```python
from build123d import *

# Parameters (mm, degrees)
SKETCH1_W           = 25.4
SKETCH1_H           = 50.8
SKETCH1_W_2         = 22.2504
SKETCH1_H_2         = 47.6504
BOSS_EXTRUDE1_DEPTH = 406.4
SKETCH2_R           = 14.2875
CUT_EXTRUDE1_DEPTH  = 51.8
SKETCH3_R           = 14.2875
SKETCH3_R_2         = 12.6365
BOSS_EXTRUDE2_DEPTH = 50.8


with BuildPart() as part:
    # Sketch1 → Boss-Extrude1 (new body)
    with BuildSketch(Plane.XY):
        Rectangle(SKETCH1_W, SKETCH1_H)
        Rectangle(SKETCH1_W_2, SKETCH1_H_2, mode=Mode.SUBTRACT)
    extrude(amount=BOSS_EXTRUDE1_DEPTH)

    # Sketch2 → Cut-Extrude1 (cut, through all)
    with BuildSketch(Plane(origin=(0, 25.4, 0), x_dir=(1, 0, 0), z_dir=(0, 1, 0))):
        Circle(SKETCH2_R)
        with Locations((0, -406.4)):
            Circle(SKETCH2_R)
    extrude(amount=-CUT_EXTRUDE1_DEPTH, mode=Mode.SUBTRACT)

    # Sketch3 → Boss-Extrude2 (add)
    with BuildSketch(Plane(origin=(0, 25.4, 0), x_dir=(1, 0, 0), z_dir=(0, 1, 0))):
        Circle(SKETCH3_R)
        Circle(SKETCH3_R_2, mode=Mode.SUBTRACT)
        with Locations((0, -406.4)):
            Circle(SKETCH3_R)
        with Locations((0, -406.4)):
            Circle(SKETCH3_R_2, mode=Mode.SUBTRACT)
    extrude(amount=-BOSS_EXTRUDE2_DEPTH)


solid = part.part
```
The model under review builds one solid part; all positions refer to its coordinate system, in mm. A direction names the side the tool comes from. Coordinates: 2 decimals unless noted, no trailing zeros. Order: outer loops, then holes, each group sorted by start corner. A loop starts at its lowest first (then second) coordinate and runs counter-clockwise, first axis right, second up. Notation, with made-up numbers: (42, -37) -> (76, -37) arc R23 ccw to (76, -18) -> close; hole circle Ø3 at (-39, -38). An arc over 180 degrees is marked (long way). Answer in a Markdown table with one row per item. Add a question column.
Item 1: Clearance check with flat-ended pins moving along their axes: pin 1 (15 mm diameter, centred on y = 12, z = 278.5, fed in from +X); pin 2 (6 mm diameter, centred on x = 11, y = -1.5, fed in from -Z); pin 3 (5 mm diameter, centred on x = -7, y = 8, fed in from -Z). State where each tip first meets the part, or that it passes through.
Item 2: We need section B-B on z = 0. Write out the cut boundary in (x, y).
Item 3: To check wall thickness, follow probe 1 along Z at (x, y) = (0.25, 11.5); probe 2 along Z at (x, y) = (1.25, 1); probe 3 along Y at (x, z) = (-7.75, 317). State the ranges of each line that lie inside material, in increasing order.
Item 4: Machinability: for faces 1 (the flat face through (3, -25.4, 200)), 2 (the flat face through (12.7, 0, 200)), 3 (the flat face through (0, 23.825, 200)), 4 (the flat face through (-12.7, 0, 200)), which of the approach directions +Z, -Z, +X, -X, +Y, -Y give a long, thin tool a straight path to every point of the face, cutting with its end or side? Answer none if there is none.
Item 5: We need section A-A on x = 0. Write out the cut boundary in (y, z), plus the area to 3 significant figures.
Item 6: We need section C-C on y = 18.5. Write out the cut boundary in (x, z) (1 decimal), plus the area to 3 significant figures.
Item 7: Mouldability with a two-part tool opening along Z and no side actions: class faces 5 (the cylindrical face through (-1.65, 0.36, 393.87)), 6 (the flat face through (3, 25.4, 200)) as +Z half, -Z half, draft (parallel to the pull), parting line (faces both ways), or undercut.
Final values:
| question | item | result |
|---|---|---|
| 1 | pin 1 | stops at x = 12.7 |
| 1 | pin 2 | stops at z = -11.84 |
| 1 | pin 3 | stops at z = -13.56 |
| 2 | outline | (-14.29, -25.4) -> (-12.64, -25.4) -> (-12.64, 25.4) -> (-14.29, 25.4) -> close; (12.64, -25.4) -> (14.29, -25.4) -> (14.29, 25.4) -> (12.64, 25.4) -> close |
| 3 | probe 1 | z = -14.29 to -12.63, 12.63 to 14.29, 392.11 to 393.77, 419.03 to 420.69 |
| 3 | probe 2 | z = -14.23 to -12.57, 12.57 to 14.23, 392.17 to 393.83, 418.97 to 420.63 |
| 3 | probe 3 | y = -25.4 to -23.83, 23.83 to 25.4 |
| 4 | face 1 | +Z, -Z, +X, -X, -Y |
| 4 | face 2 | +X, +Y, -Y |
| 4 | face 3 | none |
| 4 | face 4 | -X, +Y, -Y |
| 5 | outline | (-25.4, -14.29) -> (25.4, -14.29) -> (25.4, -12.64) -> (-25.4, -12.64) -> close; (-25.4, 12.64) -> (25.4, 12.64) -> (25.4, 393.76) -> (-25.4, 393.76) -> close; (-25.4, 419.04) -> (25.4, 419.04) -> (25.4, 420.69) -> (-25.4, 420.69) -> close; hole (-23.83, 14.29) -> (23.83, 14.29) -> (23.83, 392.11) -> (-23.83, 392.11) -> close |
| 5 | area | 1,530 mm2 |
| 6 | outline | (-12.7, 6.5) arc R14.3 ccw (long way) to (12.7, 6.5) -> (12.7, 399.9) arc R14.3 ccw (long way) to (-12.7, 399.9) -> close; hole circle Ø25.3 at (0, 0); hole circle Ø25.3 at (0, 406.4); hole (-11.1, 9) arc R14.3 cw to (11.1, 9) -> (11.1, 397.4) arc R14.3 cw to (-11.1, 397.4) -> close |
| 6 | area | 1,510 mm2 |
| 7 | face 5 | undercut |
| 7 | face 6 | draft |
